Part model, mm, in its own coordinate system. A direction names the side the tool comes from. Round coordinates to 2 decimals unless told otherwise and drop trailing zeros. Loops run counter-clockwise (first coordinate to the right, second up) from the corner with the lowest first, then second, coordinate; pieces in that order, holes last. Notation, with made-up numbers: M 32,69.5 L 63,69.5 A16 ccw 63,76.5 Z; hole C 57.25,-37.5 d9. An arc over 180 degrees is marked long. Put each result on its own line as item: value. Start each with the question number.
1) Probe line 1 along X through (y, z) = (-22.5, 31.5); line 2 along Y through (x, z) = (10.25, 29.5); line 3 along X through (y, z) = (-20.5, 29). List the from-to ranges inside material, lowest first.
2) Drop flat-ended pins along their axis: pin 1 Ø4 at (x, z) = (11, 19) entering from -Y; pin 2 Ø1.1 at (y, z) = (-19, 18.5) entering from -X; pin 3 Ø2 at (x, z) = (8, 11) entering from +Y. Give the stop position or say it passes through.
3) Slice it at B-B on y = -6. Give the cut face in (x, z), then the cut area to 3 significant figures.
4) Pull direction Z, two halves, no side cores. Call faces 1 (the flat face through (20.9, -2.26, 18.73)), 2 (the flat face through (16, -13, 0)), 3 (the cylindrical face through (8.265, -23.954, 2.686)), 4 (the flat face through (16, -13, 38)): +Z half, -Z half, draft (parallel to the pull), parting line (faces both ways), or undercut.
5) Slice it at A-A on z = 28. Give the cut face in (x, y).
6) Which spindle directions (+Z, -Z, +X, -X, +Y, -Y) get a long thin tool onto all of the face, cutting with end or side? Do faces 5 (the flat face through (9.467, -19, 19)), 6 (the cylindrical face through (26.43, 3, 2.69)). Say none if no direction does.
7) Slice it at C-C on x = 17. Give the cut face in (y, z).
```python
from build123d import *

# Parameters (mm, degrees)
BOSS_EXTRUDE1_DEPTH = 38
SKETCH2_R           = 1.85
CUT_EXTRUDE1_DEPTH  = 21.73151986


with BuildPart() as part:
    # Sketch1 → Boss-Extrude1 (new body)
    with BuildSketch(Plane.XY):
        with BuildLine():
            Line((19.245374747, -3.140947442), (22.599041108, -1.357255436))
            Line((22.599041108, -1.357255436), (27.628159729, 6.106521483))
            Line((27.628159729, 6.106521483), (28.872122548, 5.268335046))
            Line((28.872122548, 5.268335046), (5.682297797, -29.147969636))
            Line((5.682297797, -29.147969636), (4.438334977, -28.309783199))
            Line((4.438334977, -28.309783199), (9.467453598, -20.84600628))
            Line((9.467453598, -20.84600628), (9.467453598, -17.047501939))
            ThreePointArc((9.467453598, -17.047501939), (15.951636041, -11.21585073), (19.245374747, -3.140947442))
        make_face()
    extrude(amount=BOSS_EXTRUDE1_DEPTH)

    # Sketch2 → Cut-Extrude1 (cut, through all)
    with BuildSketch(Plane(origin=(16.171516658, -10.896423679, 0), x_dir=(0, 0, 1), z_dir=(-0.829308547, 0.558790958, 0))):
        with Locations((4.05, 16.002556295)):
            Circle(SKETCH2_R)
        with Locations((33.55, 16.002556295)):
            Circle(SKETCH2_R)
        with Locations((4.05, -16.497443705)):
            Circle(SKETCH2_R)
        with Locations((33.55, -16.497443705)):
            Circle(SKETCH2_R)
    extrude(amount=-CUT_EXTRUDE1_DEPTH, mode=Mode.SUBTRACT)


solid = part.part
```
Recorded:
1. line 1: x = 8.35 to 10.16
1. line 2: y = -22.37 to -16.59
1. line 3: x = 9.47 to 11.51
2. pin 1: stops at y = -24.22
2. pin 2: stops at x = 9.47
2. pin 3: stops at y = -21.54
3. outline: M 18.55,0 L 21.28,0 L 21.28,38 L 18.55,38 Z
3. area: 104 mm2
4. face 1: draft
4. face 2: -Z half
4. face 3: undercut
4. face 4: +Z half
5. outline: M 4.44,-28.31 L 5.68,-29.15 L 28.87,5.27 L 27.63,6.11 L 22.6,-1.36 L 19.25,-3.14 A19.5 cw 9.47,-17.05 L 9.47,-20.85 Z
6. face 5: +Z, -Z, -X, +Y
6. face 6: none
7. outline: M -12.35,0 L -9.55,0 L -9.55,38 L -12.35,38 Z
